Part model, mm, in its own coordinate system. Give positions to 0.01 mm unless a question says otherwise; leave off trailing zeros. Loops run counter-clockwise (first coordinate to the right, second up) from the corner with the lowest first, then second, coordinate; pieces in that order, holes last. Notation, with made-up numbers: (81.25, 16.25) -> (92.25, 16.25) arc R23 cw to (92.25, 40.25) -> close; hole circle Ø5 at (-7.5, 89). An arc over 180 degrees is marked (long way). One line per question, with ' | ' between items.
Autodesk Inventor part; units mm, degrees
ref_plane "YZ Plane" through (0, 0, 0) normal (1, 0, 0) x (0, 1, 0)
ref_plane "XZ Plane" through (0, 0, 0) normal (0, 1, 0) x (-1, 0, 0)
ref_plane "XY Plane" through (0, 0, 0) normal (0, 0, 1) x (1, 0, 0)
sketch "Sketch1" plane through (0, 0, 0) normal (0, 1, 0) x (-1, 0, 0)
  circle A0 centre (0, 0) radius 165.1
  point P0 (0, 76.2)
  point P1 (0, 101.6)
  dimension "d0" = 330.2
  dimension "d4" = 25.4
  dimension "d5" = 76.2
extrude "Extrusion1" add sketch "Sketch1" along normal blind 38.1
fillet "Fillet1" radius 12.7 1 edges at (165.1, 38.1, 0)
hole "Hole1" at (0, 0, 76.2) at (0, 0, 101.6) direction (0, 1, 0) diameter 5.6134 depth 19.05 tip angle 118
pattern_circular "Circular Pattern1" count 4 over 360 about axis through (0, -10, 0) along (0, 1, 0) of "Hole1"
properties part number "Seat" material "Wood (Birch)"
1) Drill centre lines: line 1 (X direction, y = 13.75, z = 101.6); line 2 (Z direction, x = -23, y = 10.5); line 3 (Z direction, x = 143.5, y = 25.5). Where is each one in solid material? Low to high.
Found:
line 1: -130.14 to -2.81, 2.81 to 130.14 | line 2: -163.49 to 163.49 | line 3: -81.64 to 81.64
2) Pin check, flat tips, straight feed: P1, Ø2, axis at y = 20, z = -58, coming from the -X side; P2, Ø1.5, axis at y = 6.5, z = 41.5, coming from the -X side; P3, Ø3.5, axis at x = 0, z = 101.6, coming from the -Y side. Stop position of each tip, or through.
Found:
P1: x = -154.95 | P2: x = -159.99 | P3: y = 19.68
3) Saw through at B-B (y = 31.5). Give the cut face in (x, z).
Found:
outline: circle Ø327.08 at (0, 0)
4) Saw through at A-A (y = 6). State how many separate pieces and enclosed holes the cut face has, and give its area (3 significant figures).
Found:
separate pieces: 1 | enclosed holes: 8 | area: 85,400 mm2
